```python
from build123d import *

# Parameters (mm, degrees)
SKETCH3_W           = 76.2
SKETCH3_H           = 76.2
BOSS_EXTRUDE1_DEPTH = 109.22
SKETCH4_W           = 33.655
SKETCH4_H           = 69.85
CUT_EXTRUDE2_DEPTH  = 101.6
FILLET10_R          = 1.27


with BuildPart() as part:
    # Sketch3 → Boss-Extrude1 (new body)
    with BuildSketch(Plane(origin=(0, 0, 0), x_dir=(1, 0, 0), z_dir=(0, 1, 0))):
        with Locations((-125.900159602, -33.824710809)):
            Rectangle(SKETCH3_W, SKETCH3_H)
    extrude(amount=BOSS_EXTRUDE1_DEPTH)

    # Sketch4 → Cut-Extrude2 (cut)
    with BuildSketch(Plane(origin=(0, 109.22, 0), x_dir=(1, 0, 0), z_dir=(0, 1, 0))):
        with Locations((-143.997659602, -33.824710809)):
            Rectangle(SKETCH4_W, SKETCH4_H)
        with Locations((-107.802659602, -33.824710809)):
            Rectangle(SKETCH4_W, SKETCH4_H)
    extrude(amount=-CUT_EXTRUDE2_DEPTH, mode=Mode.SUBTRACT)

    # Fillet10
    fillet10_edges = [part.edges().sort_by_distance(p)[0] for p in [
        (-87.800159602, 109.22, 33.824710809),
        (-125.900159602, 109.22, -4.275289191),
        (-124.630159602, 7.62, 33.824710809),
        (-164.000159602, 109.22, 33.824710809),
        (-125.900159602, 0, -4.275289191),
        (-87.800159602, 0, 33.824710809),
        (-125.900159602, 0, 71.924710809),
        (-164.000159602, 0, 33.824710809),
        (-164.000159602, 54.61, -4.275289191),
        (-87.800159602, 54.61, -4.275289191),
        (-87.800159602, 54.61, 71.924710809),
        (-164.000159602, 54.61, 71.924710809),
        (-125.900159602, 109.22, 71.924710809),
    ]]
    fillet(fillet10_edges, radius=FILLET10_R)


solid = part.part
```
The listing builds one solid part. Answer for the finished solid, in the listing's coordinates (mm). A direction names the side the tool comes from. Give positions to 0.01 mm unless a question says otherwise; leave off trailing zeros. Order: outer loops, then holes, each group sorted by start corner. A loop starts at its lowest first (then second) coordinate and runs counter-clockwise, first axis right, second up. Notation, with made-up numbers: (74, 34) - (105, 34) arc R6 ccw to (105, 40) - close; hole circle Ø2 at (12.25, 62.5). An arc over 180 degrees is marked (long way). Use one line per item in the form item = value. Start each with the question number.
(1) Consider line 1 (X direction, y = 95.5, z = 34.5); line 2 (Z direction, x = -158.5, y = 20.5); line 3 (Y direction, x = -107, z = 23). Determine where each line is inside the solid, lowest interval first. Write a range as from..to.
(2) For faces 1 (the flat face through (-124.63, 60, 34)), 2 (the flat face through (-126, 109.22, 34)), determine the directions among +Z, -Z, +X, -X, +Y, -Y from which every point of the face is accessible in a straight line to the end or side of a thin tool.
(3) A cutting plane is placed at B-B, the plane x = -158.5. Write down the section's boundary in (y, z).
(4) A cutting plane is placed at C-C, the plane z = 13.5. Write down the section's boundary in (x, y), then the cut area to 3 significant figures.
(5) A flat-ended cylindrical pin translates along its axis: pin 1 Ø10 at (x, z) = (-143.5, 22) entering from +Y. Find the tip coordinate at first contact, or state that the pin passes through.
(6) The mould has two halves that part along X. Classify faces 3 (the flat face through (-126, 54, 71.925)), 4 (the flat face through (-127.17, 59, 34)), 5 (the flat face through (-164, 54, 34)): released by +X, released by -X, zero draft, split by the parting line, or undercut.
(7) A cutting plane is placed at A-A, the plane y = 35. Write down the section's boundary in (x, z).
Ans:
q1.line_1 = -164..-160.83, -127.17..-124.63, -90.98..-87.8
q1.line_2 = -4.28..-1.1, 68.75..71.92
q1.line_3 = 0..7.62
q2.face_1 = +Y
q2.face_2 = +Z, -Z, +X, -X, +Y
q3.outline = (0, -3.01) arc R1.27 ccw to (1.27, -4.28) - (107.95, -4.28) arc R1.27 ccw to (109.22, -3.01) - (109.22, -1.1) - (7.62, -1.1) - (7.62, 68.75) - (109.22, 68.75) - (109.22, 70.65) arc R1.27 ccw to (107.95, 71.92) - (1.27, 71.92) arc R1.27 ccw to (0, 70.65) - close
q4.outline = (-164, 1.27) arc R1.27 ccw to (-162.73, 0) - (-89.07, 0) arc R1.27 ccw to (-87.8, 1.27) - (-87.8, 107.95) arc R1.27 ccw to (-89.07, 109.22) - (-90.98, 109.22) - (-90.98, 7.62) - (-123.36, 7.62) arc R1.27 cw to (-124.63, 8.89) - (-124.63, 109.22) - (-127.17, 109.22) - (-127.17, 7.62) - (-160.83, 7.62) - (-160.83, 109.22) - (-162.73, 109.22) arc R1.27 ccw to (-164, 107.95) - close
q4.area = 1,480 mm^2
q5.pin_1 = 7.62
q6.face_3 = zero draft
q6.face_4 = undercut
q6.face_5 = released by -X
q7.outline = (-164, -3.01) arc R1.27 ccw to (-162.73, -4.28) - (-89.07, -4.28) arc R1.27 ccw to (-87.8, -3.01) - (-87.8, 70.65) arc R1.27 ccw to (-89.07, 71.92) - (-162.73, 71.92) arc R1.27 ccw to (-164, 70.65) - close; hole (-160.83, -1.1) - (-127.17, -1.1) - (-127.17, 68.75) - (-160.83, 68.75) - close; hole (-124.63, -1.1) - (-90.98, -1.1) - (-90.98, 68.75) - (-124.63, 68.75) - close
